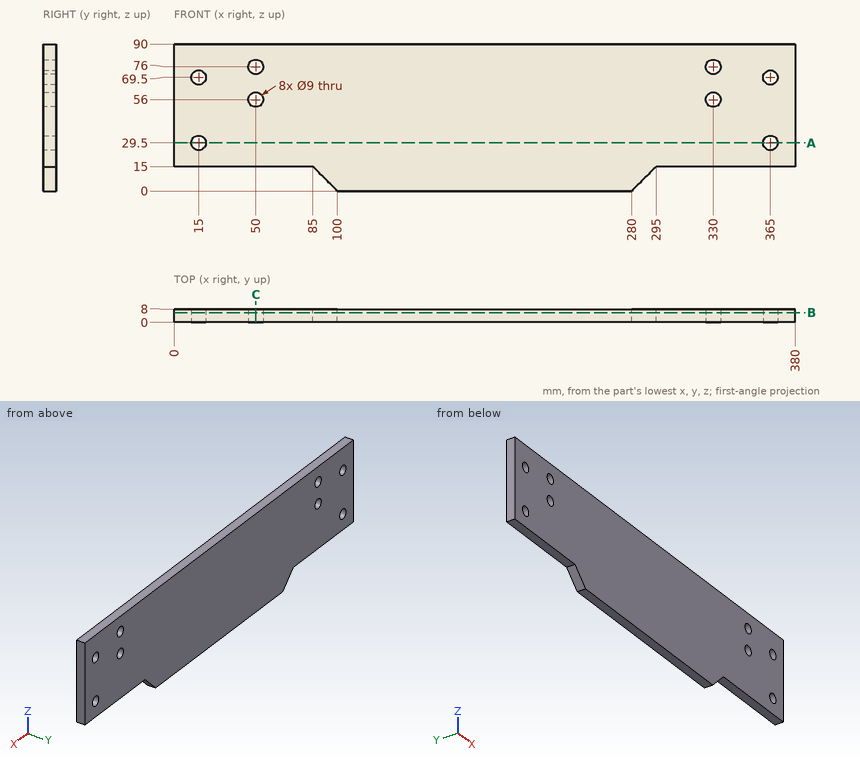
Part print with two shaded views. Sizes in mm from the minimum x, y, z corner. Coordinates: 2 decimals unless noted, no trailing zeros. Write each loop counter-clockwise with the first axis right and the second up, starting at its lowest first coordinate (ties: lowest second). Pieces come first, ordered by that corner, then holes.
(1) Drill centre lines: line 1 (X direction, y = 4.5, z = 76); line 2 (Z direction, x = 15, y = 4.75); line 3 (X direction, y = 2.25, z = 69.5). Where is each one in solid material? Low to high.
(2) Cut at B-B on y = 5.75. State how many separate pieces and enclosed holes the cut face has, and give its area (3 significant figures).
(3) Pin check, flat tip, straight feed: pin 1 Ø2.5 at (x, y) = (351.5, 4) entering from -Z. Stop position of the tip, or through.
(4) Cut at A-A on z = 29.5. List the corners of the cut face in (x, y), and give its area (3 significant figures).
(5) Cut at C-C on x = 50. List the corners of the cut face in (y, z), and give its area (3 significant figures).
Working result:
1. line 1: x = 0 to 45.5, 54.5 to 325.5, 334.5 to 380
1. line 2: z = 15 to 25, 34 to 65, 74 to 90
1. line 3: x = 0 to 10.5, 19.5 to 360.5, 369.5 to 380
2. separate pieces: 1
2. enclosed holes: 8
2. area: 30,900 mm2
3. pin 1: stops at z = 15
4. outline: (0, 0) - (10.5, 0) - (10.5, 8) - (0, 8) - close; (19.5, 0) - (360.5, 0) - (360.5, 8) - (19.5, 8) - close; (369.5, 0) - (380, 0) - (380, 8) - (369.5, 8) - close
4. area: 2,900 mm2
5. outline: (0, 15) - (8, 15) - (8, 51.5) - (0, 51.5) - close; (0, 60.5) - (8, 60.5) - (8, 71.5) - (0, 71.5) - close; (0, 80.5) - (8, 80.5) - (8, 90) - (0, 90) - close
5. area: 456 mm2
